Autodesk Inventor part; units mm, degrees
ref_plane "YZ Plane" through (0, 0, 0) normal (1, 0, 0) x (0, 1, 0)
ref_plane "XZ Plane" through (0, 0, 0) normal (0, 1, 0) x (-1, 0, 0)
ref_plane "XY Plane" through (0, 0, 0) normal (0, 0, 1) x (1, 0, 0)
ref_plane "Arbeitsebene1" through (0, 0, 0) normal (0, 0, 1) x (1, 0, 0)
sketch "Skizze1" plane through (0, 0, 0) normal (0, 0, 1) x (1, 0, 0)
  line L0 (8.8004, 63) -> (20, 63)
  line L1 (20, 63) -> (20, 53)
  line L2 (8.8004, 63) -> (-10, 63)
  line L3 (-10, 63) -> (-10, 53)
  line L4 (-10, 53) -> (20, 53)
  circle A0 centre (-3.9345, 60.036) radius 1.4
  circle A1 centre (11.0655, 60.036) radius 1.4
  line L5 (-10, 63) -> (20, 63)
  line L6 (20, 63) -> (20, 68)
  line L7 (20, 68) -> (-10, 68)
  line L8 (-10, 68) -> (-10, 63)
  point P0 (12.8, 45.75)
  point P1 (12.8, 36.25)
  dimension "d11" = 30
  dimension "d14" = 10
  dimension "d16" = 2.8
  dimension "d17" = 2.8
  dimension "d18" = 15
  dimension "d19" = 0
  dimension "d20" = 5
extrude "Extrusion1" add sketch "Skizze1" along normal blind 5
sketch "Skizze4" plane through (0, 0, 5) normal (0, 0, 1) x (1, 0, 0)
  line L0 (20, 68) -> (-10, 68)
  line L1 (-10, 68) -> (-10, 53)
  line L2 (-10, 53) -> (20, 53)
  circle A0 centre (-3.9345, 60.036) radius 1.4
  circle A1 centre (11.0655, 60.036) radius 1.4
  line L3 (-1.6845, 57.3969) -> (8.8155, 57.3969)
  line L4 (8.8155, 57.3969) -> (8.8155, 70.8506)
  line L5 (8.8155, 70.8506) -> (-1.6845, 70.8506)
  line L6 (-1.6845, 70.8506) -> (-1.6845, 57.3969)
  line L7 (20, 53) -> (20, 68)
  point P0 (0, 0)
  point P1 (8.8155, 68)
  point P2 (-1.6845, 68)
  dimension "d21" = 10.5
  dimension "d22" = 2.25
extrude "Extrusion3" cut sketch "Skizze4" against normal blind 5 contours L4 L3 L6 L0
sketch "Skizze5" plane through (0, 0, 5) normal (0, 0, 1) x (1, 0, 0)
  line L0 (-1.6845, 57.3969) -> (-1.6845, 68)
  line L1 (-1.6845, 68) -> (-10, 68)
  line L2 (-10, 68) -> (-10, 53)
  line L3 (-10, 53) -> (20, 53)
  line L4 (20, 53) -> (20, 68)
  line L5 (20, 68) -> (8.8155, 68)
  line L6 (8.8155, 68) -> (8.8155, 57.3969)
  line L7 (8.8155, 57.3969) -> (-1.6845, 57.3969)
  circle A0 centre (11.0655, 60.036) radius 1.4
  circle A1 centre (-3.9345, 60.036) radius 1.4
  line L8 (-1.6845, 53) -> (-10, 53)
  line L9 (-10, 53) -> (-10, 113)
  line L10 (-10, 113) -> (-1.6845, 113)
  line L11 (-1.6845, 113) -> (-1.6845, 53)
  circle A2 centre (-5.8422, 84) radius 1.6
  circle A3 centre (-5.8422, 104) radius 1.6
  point P0 (0, 0)
  dimension "d26" = 45
  dimension "d27" = 3.2
  dimension "d28" = 3.2
  dimension "d29" = 20
  dimension "d30" = 16
extrude "Extrusion4" add sketch "Skizze5" along normal blind 8
sketch "Skizze6" plane through (0, 0, 5) normal (0, 0, -1) x (-1, 0, 0)
  line L0 (1.6845, 68) -> (10, 68)
  line L1 (10, 113) -> (10, 68)
  line L2 (1.6845, 113) -> (10, 113)
  line L3 (1.6845, 68) -> (1.6845, 113)
  circle A0 centre (5.8422, 104) radius 1.6
  circle A1 centre (5.8422, 84) radius 1.6
  line L4 (1.6845, 68) -> (10, 68)
  line L5 (10, 68) -> (10, 113)
  line L6 (10, 113) -> (1.6845, 113)
  line L7 (1.6845, 113) -> (1.6845, 68)
  point P0 (0, 0)
extrude "Extrusion5" cut sketch "Skizze6" against normal blind 3
properties part number "30_XYTable_Aliexpress_naked_endstopX_adapter"
Can you work these out from the model? Positions are in its coordinate system, mm. A direction names the side the tool comes from. Give positions to 0.01 mm unless a question says otherwise; leave off trailing zeros. Write each loop counter-clockwise with the first axis right and the second up, starting at its lowest first coordinate (ties: lowest second). Pieces come first, ordered by that corner, then holes. Notation, with made-up numbers: (-20.75, -4) -> (-7.75, -4) arc R10 ccw to (-7.75, 8) -> close; hole circle Ø8 at (24.25, 21). An arc over 180 degrees is marked (long way). One line per item, written item: value.
Q1. For P1, Ø3, axis at x = 6, z = 5.5, coming from the +Y side; P2, Ø4, axis at x = -8, y = 80, coming from the -Z side, each with a flat end and sliding along its axis, tell me the tip position at first contact or that it passes through.
Results found:
P1: stops at y = 57.4
P2: stops at z = 8
Q2. Imagine slicing it at B-B on x = 11.25. Please give me the cut outline in (y, z).
Results found:
outline: (53, 0) -> (58.65, 0) -> (58.65, 13) -> (53, 13) -> close; (61.42, 0) -> (68, 0) -> (68, 13) -> (61.42, 13) -> close
Q3. Imagine slicing it at A-A on y = 62.5. Please give me the cut outline in (x, z).
Results found:
outline: (-10, 0) -> (-1.68, 0) -> (-1.68, 13) -> (-10, 13) -> close; (8.82, 0) -> (20, 0) -> (20, 13) -> (8.82, 13) -> close
Q4. Please list where these lines run through material, in increasing order: line 1 (X direction, y = 58.5, z = 3.25); line 2 (X direction, y = 84, z = 10.45); line 3 (X direction, y = 92, z = 9.5). Write a range as [from, to].
Results found:
line 1: x = [-10, -1.68], [8.82, 20]
line 2: x = [-10, -7.44], [-4.24, -1.68]
line 3: x = [-10, -1.68]
Q5. Imagine slicing it at D-D on y = 72. Please give me the cut outline in (x, z).
Results found:
outline: (-10, 8) -> (-1.68, 8) -> (-1.68, 13) -> (-10, 13) -> close
Q6. We'd pull the mould along X, two halves only. Please class faces 1 (the face through (-10, 77, 9)), 2 (the face through (8.816, 63, 7)), 3 (the face through (-6.05, 82.414, 10.465)), 4 (the face through (-6, 68, 4)): +X half, -X half, draft (parallel to the pull), parting line (faces both ways), or undercut.
Results found:
face 1: -X half
face 2: undercut
face 3: undercut
face 4: draft
Q7. Which directions (+Z, -Z, +X, -X, +Y, -Y) give clear straight access to the entire face, cutting with the end or side of a thin tool? Please do faces 5 (the face through (-6, 113, 10)), 6 (the face through (-6, 91, 8)), 7 (the face through (14, 68, 6)), 8 (the face through (-1.684, 79, 9)).
Results found:
face 5: +Z, -Z, +X, -X, +Y
face 6: -Z, +X, -X, +Y
face 7: +Z, -Z, +X, +Y
face 8: +Z, -Z, +Y
Q8. Imagine slicing it at C-C on z = 5.5. Please give me the cut outline in (x, y), and give its area (3 significant figures).
Results found:
outline: (-10, 53) -> (20, 53) -> (20, 68) -> (8.82, 68) -> (8.82, 57.4) -> (-1.68, 57.4) -> (-1.68, 68) -> (-10, 68) -> close; hole circle Ø2.8 at (-3.93, 60.04); hole circle Ø2.8 at (11.07, 60.04)
area: 326 mm^2
